from build123d import *

# Parameters (mm, degrees)
F1_DEPTH      = 203.2
F1_DEPTH_BACK = 203.2
F4_DEPTH      = 406.4
F5_R          = 6.35
F6_DEPTH      = 406.4


# Not quite as in the source:
# - a feature names something its author has since deleted; it is built from what else it names


with BuildPart() as f1:
    # F0 (on Front) → F1 (new body, two sides)
    with BuildSketch(Plane.XZ) as f1_sk:
        with BuildLine():
            Line((203.2, 0), (12.7, 0))
            ThreePointArc((12.7, 0), (0, -12.7), (-12.7, 0))
            Line((-12.7, 0), (-203.2, 0))
            Line((-203.2, 0), (-203.2, -228.6))
            Line((-203.2, -228.6), (203.2, -228.6))
            Line((203.2, -228.6), (203.2, 0))
        make_face()
        with BuildLine():
            Line((12.7, 0), (6.35, 0))
            ThreePointArc((6.35, 0), (0, -6.35), (-6.35, 0))
            Line((-6.35, 0), (-12.7, 0))
            ThreePointArc((-12.7, 0), (0, -12.7), (12.7, 0))
        make_face()
        with BuildLine():
            ThreePointArc((-6.35, 0), (0, 6.35), (6.35, 0))
            Line((6.35, 0), (12.7, 0))
            ThreePointArc((12.7, 0), (0, 12.7), (-12.7, 0))
            Line((-12.7, 0), (-6.35, 0))
        make_face()
    extrude(amount=F1_DEPTH)
    extrude(f1_sk.sketch, amount=-F1_DEPTH_BACK)

    # F3 (on face) → F4 (join)
    with BuildSketch(Plane.YZ.offset(203.2)):
        with BuildLine():
            Line((-12.7, 0), (12.7, 0))
            ThreePointArc((12.7, 0), (0, 12.7), (-12.7, 0))
        make_face()
        with BuildLine():
            ThreePointArc((-12.7, 0), (0, -12.7), (12.7, 0))
            Line((12.7, 0), (-12.7, 0))
        make_face()
    extrude(amount=-F4_DEPTH)

    # F5 (on face) → F6 (cut)
    with BuildSketch(Plane.YZ.offset(203.2)):
        Circle(F5_R)
    extrude(amount=-F6_DEPTH, mode=Mode.SUBTRACT)

    # F2 (on Front) → F7 (revolve, cut)
    with BuildSketch(Plane.XZ):
        with BuildLine():
            Line((0, 190.5), (0, -190.5))
            ThreePointArc((0, -190.5), (190.5, 0), (0, 190.5))
        make_face()
    revolve(axis=Axis((0, 0, 0), (0, 0, -1)), mode=Mode.SUBTRACT)


solid = f1.part
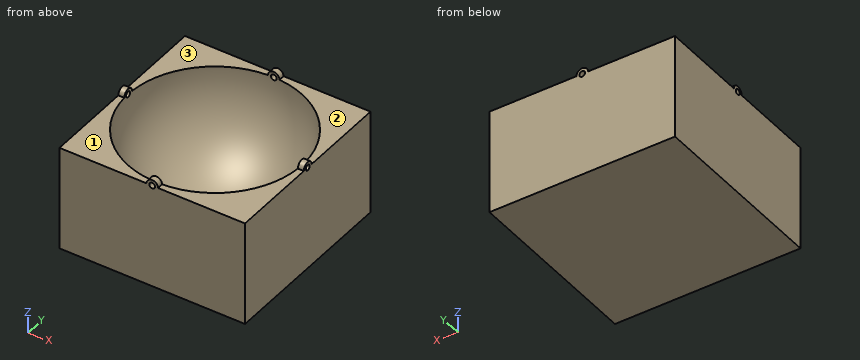
Can you work these out from the model? Positions are in its coordinate system, mm. Face numbers are marked on the shaded views. A direction names the side the tool comes from. Coordinates: 2 decimals unless noted, no trailing zeros. Order: outer loops, then holes, each group sorted by start corner. A loop starts at its lowest first (then second) coordinate and runs counter-clockwise, first axis right, second up. Notation, with made-up numbers: M -32,-20 L 3,-20 A10 cw 3,-13 Z; hole C 48.25,63 d2. An arc over 180 degrees is marked long. Write item = value, one per line.
(1) For the marked faces 1, 2 and 3, which set-ups out of +Z, -Z, +X, -X, +Y, -Y let a thin tool reach every point of the face, with its end or its side?
Results are:
face_1 = +Z, -X, -Y
face_2 = +Z, +X, +Y
face_3 = +Z, -X, +Y
(2) Suppose I cut it at D-D on x = -160. Please give me the cut outline in (y, z).
Results are:
outline = M -203.2,-228.6 L 203.2,-228.6 L 203.2,0 L 103.39,0 A103.39 cw -103.39,0 L -203.2,0 Z
(3) For pin 1 Ø12 at (x, y) = (8, -64.5) entering from +Z; pin 2 Ø11.5 at (x, z) = (0, 0) entering from -Y; pin 3 Ø6 at (x, y) = (136.5, 94.5) entering from +Z, each with a flat end and sliding along its axis, tell me the tip position at first contact or that it passes through.
Results are:
pin_1 = -176.78
pin_2 = through
pin_3 = -87.88
(4) Suppose I cut it at A-A on y = 0. Please give me the cut outline in (x, z), plus the area to 3 significant figures.
Results are:
outline = M -203.2,-228.6 L 203.2,-228.6 L 203.2,-6.35 L 190.39,-6.35 A190.5 cw -190.39,-6.35 L -203.2,-6.35 Z; M -203.2,6.35 L -190.39,6.35 A190.5 cw -190.08,12.7 L -203.2,12.7 Z; M 190.08,12.7 A190.5 cw 190.39,6.35 L 203.2,6.35 L 203.2,12.7 Z
area = 35,900 mm2
(5) Suppose I cut it at C-C on z = -133.5. Please give me the cut outline in (x, y).
Results are:
outline = M -203.2,-203.2 L 203.2,-203.2 L 203.2,203.2 L -203.2,203.2 Z; hole C 0,0 d271.79
(6) I need wall thicknesses on line 1 along Z through (x, y) = (-197.25, 0); line 2 along Z through (x, y) = (186, -148); line 3 along Y through (x, z) = (22.5, -117). Which ranges of each line are inside material? Lowest first, please. Write a range as [from, to].
Results are:
line_1 = [-228.6, -6.35], [6.35, 12.7]
line_2 = [-228.6, 0]
line_3 = [-203.2, -148.64], [148.64, 203.2]
